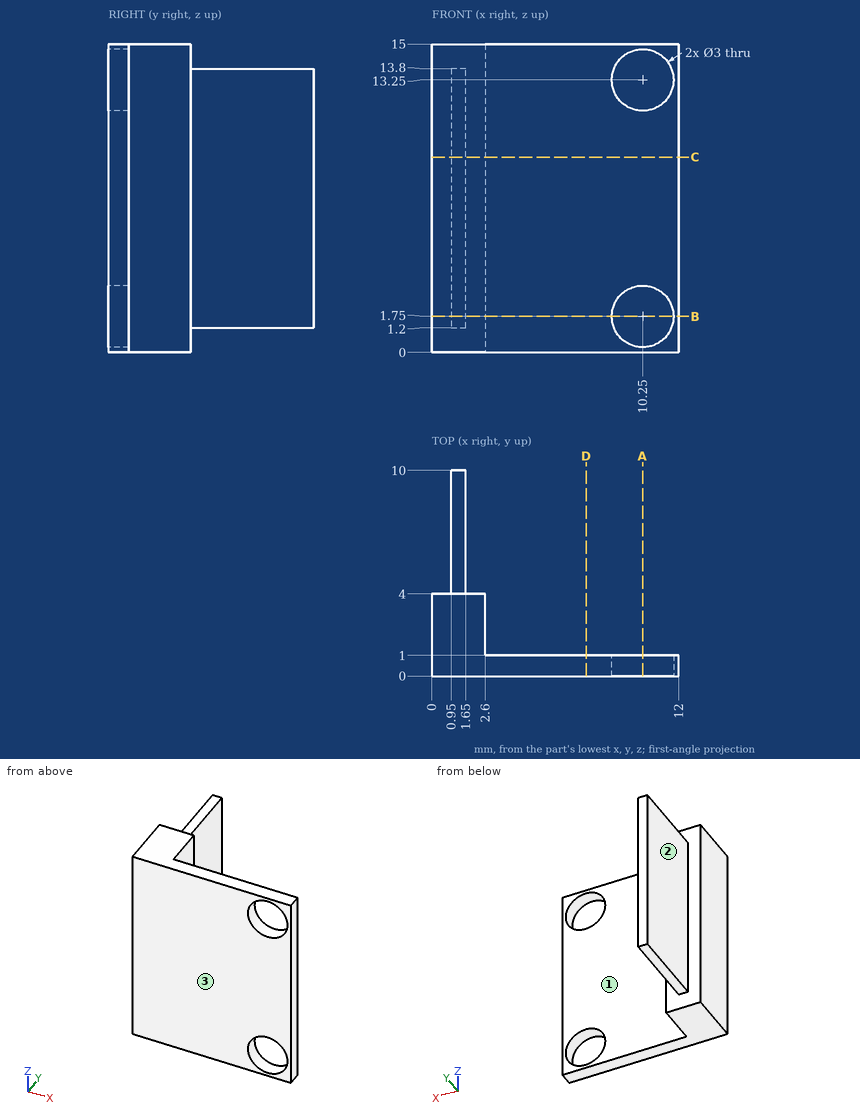
Geometry check sheet. Reference: drawing and pictorial views, mm from the part's lowest x, y, z. A direction names the side the tool comes from. Give positions to 0.01 mm unless a question says otherwise; leave off trailing zeros. Order: outer loops, then holes, each group sorted by start corner. A loop starts at its lowest first (then second) coordinate and runs counter-clockwise, first axis right, second up.
1. Access from +Z, -Z, +X, -X, +Y, -Y to the whole of each face (thin tool, end or side, straight path). Record for the marked faces 1, 2 and 3.
2. Section check A-A, the plane x = 10.25. Enter the section's corners in (y, z), and give its area (3 significant figures).
3. Section check B-B, the plane z = 1.75. Enter the section's corners in (x, y), and give its area (3 significant figures).
4. Section check C-C, the plane z = 9.5. Enter the section's corners in (x, y), and give its area (3 significant figures).
5. Gauge pin test, flat ends, axial feed: pin 1 Ø1.5 at (y, z) = (8, 9.5) entering from -X; pin 2 Ø4 at (y, z) = (7.5, 6) entering from +X; pin 3 Ø1.8 at (x, z) = (10.25, 1.75) entering from +Y; pin 4 Ø2 at (x, z) = (4, 8.5) entering from +Y. Record the tip position at first contact, or that the pin passes through.
6. Thickness scan on L1, parallel to Z at x = 10.25, y = 0.65; L2, parallel to Y at x = 6.5, z = 8.25; L3, parallel to Z at x = 1, y = 4.5. Record the ranges inside material, lowest first.
7. Section check D-D, the plane x = 7.5. Enter the section's corners in (y, z).
Values follow:
1. face 1: +Z, -Z, +X, +Y
1. face 2: +Z, -Z, -X, +Y
1. face 3: +Z, -Z, +X, -X, -Y
2. outline: (0, 0) - (1, 0) - (1, 0.25) - (0, 0.25) - close; (0, 3.25) - (1, 3.25) - (1, 11.75) - (0, 11.75) - close; (0, 14.75) - (1, 14.75) - (1, 15) - (0, 15) - close
2. area: 9.00 mm2
3. outline: (0, 0) - (8.75, 0) - (8.75, 1) - (2.6, 1) - (2.6, 4) - (1.65, 4) - (1.65, 10) - (0.95, 10) - (0.95, 4) - (0, 4) - close; (11.75, 0) - (12, 0) - (12, 1) - (11.75, 1) - close
3. area: 21.0 mm2
4. outline: (0, 0) - (12, 0) - (12, 1) - (2.6, 1) - (2.6, 4) - (1.65, 4) - (1.65, 10) - (0.95, 10) - (0.95, 4) - (0, 4) - close
4. area: 24.0 mm2
5. pin 1: stops at x = 0.95
5. pin 2: stops at x = 1.65
5. pin 3: passes through
5. pin 4: stops at y = 1
6. L1: z = 0 to 0.25, 3.25 to 11.75, 14.75 to 15
6. L2: y = 0 to 1
6. L3: z = 1.2 to 13.8
7. outline: (0, 0) - (1, 0) - (1, 15) - (0, 15) - close
